The drawing under review shows one solid part. Ordinate dimensions are in mm from its lowest x, y, z. A direction names the side the tool comes from. Give positions to 0.01 mm unless a question says otherwise; leave off trailing zeros. Order: outer loops, then holes, each group sorted by start corner. A loop starts at its lowest first (then second) coordinate and runs counter-clockwise, first axis right, second up. Notation, with made-up numbers: (-37, 39) - (1, 39) arc R15 ccw to (1, 68) - close; hole circle Ø1 at (21, 76.25). An arc over 180 degrees is marked (long way). Use CSV: the item, a comma, the result in double quotes.
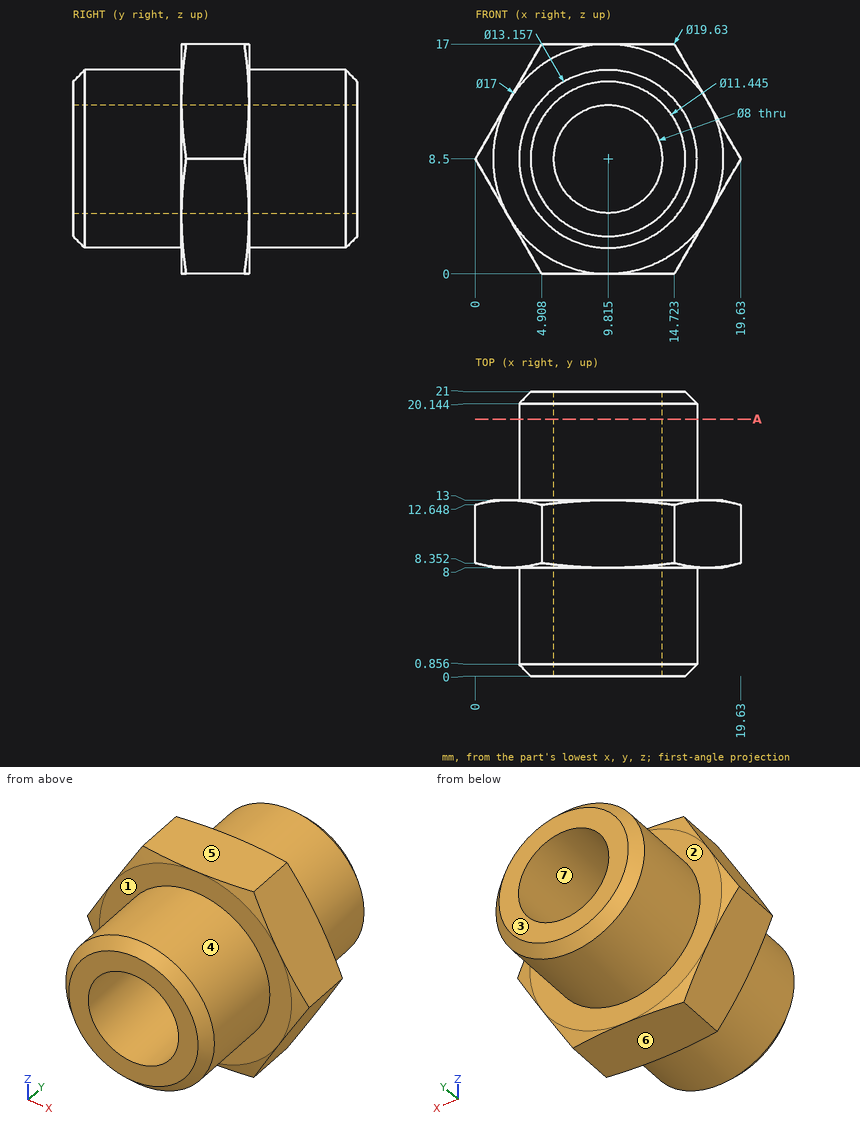
Item 1: Wall thickness on L1, parallel to Y at x = 13.5, z = 1.5; L2, parallel to Z at x = 10.75, y = 1.75; L3, parallel to X at y = 16, z = 8 (1 decimal): over which ranges is each line inside the solid? List them lowest first.
Results list:
L1,"y = 8 to 13"
L2,"z = 1.99 to 4.61, 12.39 to 15.01"
L3,"x = 3.3 to 5.8, 13.8 to 16.4"
Item 2: Clearance check with flat-ended pins moving along their axes: pin 1 (1.5 mm diameter, centred on x = 4, z = 3.5, fed in from -Y); pin 2 (1.5 mm diameter, centred on x = 5.5, y = 18, fed in from -Z); pin 3 (4 mm diameter, centred on y = 13.5, z = 12, fed in from -X). State where each tip first meets the part, or that it passes through.
Results list:
pin 1,"stops at y = 8"
pin 2,"stops at z = 2.97"
pin 3,"stops at x = 0.93"
Item 3: Mouldability with a two-part tool opening along Z and no side actions: class the marked faces 4, 5, 6 and 7 as pulls with the +Z half, pulls with the -Z half, needs draft (parallel to the pull), parting line crosses it, or undercut.
Results list:
face 4,"parting line crosses it"
face 5,"pulls with the +Z half"
face 6,"pulls with the -Z half"
face 7,"undercut"
Item 4: Take a section at A-A, the plane y = 19. Give the boundary of the cut face in (x, z) (1 decimal).
Results list:
outline,"circle Ø13.2 at (9.8, 8.5); hole circle Ø8 at (9.8, 8.5)"
Item 5: Tool access review of the marked faces 1, 2 and 3: name each direction out of +Z, -Z, +X, -X, +Y, -Y from which nothing blocks a thin tool from reaching the whole face with its end or side.
Results list:
face 1,"-Y"
face 2,"+Y"
face 3,"+Z, -Z, +X, -X, +Y"
